Geometry: final body of the model. Coordinates: model frame, mm. A direction names the side the tool comes from. Give positions to 0.01 mm unless a question says otherwise; leave off trailing zeros. Loops run counter-clockwise (first coordinate to the right, second up) from the corner with the lowest first, then second, coordinate; pieces in that order, holes last. Notation, with made-up numbers: (75.25, 70) -> (101.25, 70) arc R19 cw to (101.25, 82) -> close; hole circle Ø8 at (24, 45.25). An arc over 180 degrees is marked (long way). One line per question, with ' | ' between items. Start each with the question number.
Item 1: Set-up query: faces 4 (the flat face through (21.2, 2, 1)), 5 (the flat face through (26, 20, 1)), 6 (the flat face through (28, 0, 1)). Return all of +Z, -Z, +X, -X, +Y, -Y with unobstructed straight access to the full face (end or side cutting, diameter ignored); none if empty.
Item 2: Section D-D on x = 7.5. Return loops of the section in (y, z), then the cut area to 3 significant figures.
Item 3: Section A-A on y = 3. Return loops of the section in (x, z), then the cut area to 3 significant figures.
Item 4: Mould query, pull axis X, two halves, no side actions, for faces 1 (the flat face through (0, 14, 1)), 2 (the flat face through (9, 19, 1)), 3 (the flat face through (13, 11, 2.2)). Classes: released by +X, released by -X, zero draft, split by the parting line, or undercut.
Item 5: Section B-B on z = 0.85. Return loops of the section in (x, y), then the cut area to 3 significant figures.
Item 6: Section C-C on y = 12.5. Return loops of the section in (x, z).
Item 7: Material intervals for line 1 along X through (y, z) = (1, 1.4); line 2 along X through (y, z) = (20.5, 1.25); line 3 along Y through (x, z) = (10, 1), sorted ascending. Write a range as [from, to].
from build123d import *

# Parameters (mm, degrees)
BOSS_EXTRUDE1_DEPTH = 2.2


with BuildPart() as part:
    # Sketch1 → Boss-Extrude1 (new body)
    with BuildSketch(Plane.XY):
        with BuildLine():
            Line((17, 11), (0, 28))
            Line((0, 28), (0, 0))
            Line((0, 0), (12.8, 0))
            Line((12.8, 0), (12.8, 4.4))
            ThreePointArc((12.8, 4.4), (17, 8.6), (21.2, 4.4))
            Line((21.2, 4.4), (21.2, 0))
            Line((21.2, 0), (34, 0))
            Line((34, 0), (34, 28))
            Line((34, 28), (17, 11))
        make_face()
    extrude(amount=BOSS_EXTRUDE1_DEPTH)


solid = part.part
Result sheet:
1) face 4: +Z, -Z, -Y | face 5: +Z, -Z, +Y | face 6: +Z, -Z, +X, -X, -Y
2) outline: (0, 0) -> (20.5, 0) -> (20.5, 2.2) -> (0, 2.2) -> close | area: 45.1 mm²
3) outline: (0, 0) -> (12.8, 0) -> (12.8, 2.2) -> (0, 2.2) -> close; (21.2, 0) -> (34, 0) -> (34, 2.2) -> (21.2, 2.2) -> close | area: 56.3 mm²
4) face 1: released by -X | face 2: undercut | face 3: zero draft
5) outline: (0, 0) -> (12.8, 0) -> (12.8, 4.4) arc R4.2 cw to (21.2, 4.4) -> (21.2, 0) -> (34, 0) -> (34, 28) -> (17, 11) -> (0, 28) -> close | area: 598 mm²
6) outline: (0, 0) -> (15.5, 0) -> (15.5, 2.2) -> (0, 2.2) -> close; (18.5, 0) -> (34, 0) -> (34, 2.2) -> (18.5, 2.2) -> close
7) line 1: x = [0, 12.8], [21.2, 34] | line 2: x = [0, 7.5], [26.5, 34] | line 3: y = [0, 18]
